The listing builds one solid part. Answer for the finished solid, in the listing's coordinates (mm). A direction names the side the tool comes from. Coordinates: 2 decimals unless noted, no trailing zeros. Loops run counter-clockwise (first coordinate to the right, second up) from the corner with the lowest first, then second, coordinate; pieces in that order, holes last. Notation, with made-up numbers: M -7,-21.75 L 17,-21.75 A9 ccw 17,-14.75 Z; hole C 14.25,75.5 d2. An arc over 180 degrees is marked long. Answer as a JSON object with one key per item and string values. Group by question number.
1. A cutting plane is placed at C-C on z = -26.1. Give the vertices of the cut face in (x, y), and give its area (3 significant figures).
2. Determine the mould class of faces 1 (the face through (-4, 1, -20.6)), 2 (the face through (7, 3.95, -26)), 3 (the face through (-20.45, 7.89, -25.22)) for opening direction Z: released by +Z, released by -Z, zero draft, split by the parting line, or undercut.
3. A cutting plane is placed at B-B on z = -19.5. Give the vertices of the cut face in (x, y), and give its area (3 significant figures).
4. A cutting plane is placed at A-A on x = -21.6. Give the vertices of the cut face in (y, z).
5. For faces 4 (the face through (-7.45, 6.43, -15.73)), 5 (the face through (32.72, 7.55, -7.22)), 6 (the face through (-14.071, 3, -9)), 7 (the face through (-4, -2.85, -16)), determine the directions among +Z, -Z, +X, -X, +Y, -Y from which every point of the face is accessible in a straight line to the end or side of a thin tool.
6. A cutting plane is placed at D-D on y = -1.5. Give the vertices of the cut face in (x, z), and give its area (3 significant figures).
7. Straight lines are drawn through the part: L1, parallel to Z at x = -4, y = 8.75; L2, parallel to X at y = 4, z = -9; L3, parallel to Z at x = -21.6, y = 6.25. For each, find the intervals that lie inside material, in ascending order.
8. Given pin 1 (2.5 mm diameter, centred on x = -6.5, z = -28.5, fed in from -Y); pin 2 (2 mm diameter, centred on x = -7.5, y = 1, fed in from -Z); pin 3 (11 mm diameter, centred on x = -12, z = -17, fed in from -Y), each flat-ended and moving along its own axis, determine where each tip first touches the part or whether it passes through.
Autodesk Inventor part; units mm, degrees
ref_plane "Arbeitsebene8" through (22.1204, -2.15, -7.2) normal (1, 0, 0) x (0, 1, 0)
ref_plane "Arbeitsebene9" through (-36.7921, -9.8415, -30.1125) normal (-0.7071, 0, 0.7071) x (0.7071, 0, 0.7071)
ref_plane "Arbeitsebene11" through (-36.7921, -9.8415, -30.1125) normal (-0.7071, 0, 0.7071) x (0.7071, 0, 0.7071)
ref_plane "Arbeitsebene6" through (18.9, 3.95, -31.1) normal (0, 1, 0) x (-1, 0, 0)
sketch "Skizze13" plane through (18.9, 3.95, -31.1) normal (0, 1, 0) x (-1, 0, 0)
  circle A0 centre (40.5, 5) radius 1.45
  line L0 (29.1796, 0.9) -> (29.1796, 0)
  line L1 (45.5, 0) -> (29.1796, 0)
  line L2 (45.5, 0) -> (45.5, 10)
  line L3 (45.5, 10) -> (29.1796, 10)
  line L4 (29.1796, 10) -> (29.1796, 6.8717)
  line L5 (29.1796, 6.8717) -> (32.9296, 6.8717)
  line L6 (32.9296, 6.8717) -> (32.9296, 0.9)
  line L7 (32.9296, 0.9) -> (29.1796, 0.9)
  line L8 (24.1796, 0) -> (24.1796, 0.9)
  line L9 (24.1796, 0.9) -> (20.4296, 0.9)
  line L10 (20.4296, 0.9) -> (20.4296, 6.8717)
  line L11 (20.4296, 6.8717) -> (24.1796, 6.8717)
  line L12 (24.1796, 6.8717) -> (24.1796, 10)
  line L13 (24.1796, 10) -> (0, 10)
  line L14 (0, 0) -> (0, 10)
  line L15 (24.1796, 0) -> (0, 0)
  circle A1 centre (14.9199, 5) radius 1.45
  circle A2 centre (5.0801, 5) radius 1.45
  line L16 (29.1796, 10) -> (24.1796, 10)
  line L17 (29.1796, 0) -> (24.1796, 0)
  line L18 (55.5, 0) -> (55.5, 10)
  line L19 (55.5, 10) -> (55.473, 10)
  line L20 (55.473, 10) -> (55.473, 40)
  line L21 (55.473, 40) -> (45.5, 40)
  line L22 (45.5, 40) -> (45.5, 20)
  line L23 (45.5, 20) -> (35.5, 20)
  line L24 (35.5, 20) -> (35.5, 10.0274)
  arc A3 (35.5, 10.0274) -> (35.527, 10) centre (40.5, 14.9264) ccw
  line L25 (45.5, 10) -> (35.527, 10)
  line L26 (45.5, 0) -> (45.5, 10)
  line L27 (45.5, 0) -> (55.5, 0)
  line L28 (52.073, 16.5) -> (52.073, 3.5)
  arc A4 (48.873, 3.5) -> (52.073, 3.5) centre (50.473, 3.5) ccw
  line L29 (48.873, 3.5) -> (48.873, 16.5)
  arc A5 (52.073, 16.5) -> (48.873, 16.5) centre (50.473, 16.5) ccw
  line L30 (48.8865, 23.1111) -> (48.8865, 36.1111)
  arc A6 (52.0865, 36.1111) -> (48.8865, 36.1111) centre (50.4865, 36.1111) ccw
  line L31 (52.0865, 36.1111) -> (52.0865, 23.1111)
  arc A7 (48.8865, 23.1111) -> (52.0865, 23.1111) centre (50.4865, 23.1111) ccw
  line L32 (-10, 0) -> (0, 0)
  line L33 (0, 10) -> (0, 0)
  line L34 (16, 10) -> (0, 10)
  line L35 (16, 10) -> (16, 20)
  line L36 (16, 20) -> (-10, 20)
  line L37 (-10, 20) -> (-10, 0)
  line L38 (-3.4, 16.5) -> (-3.4, 3.5)
  arc A8 (-6.6, 3.5) -> (-3.4, 3.5) centre (-5, 3.5) ccw
  line L39 (-6.6, 3.5) -> (-6.6, 16.5)
  arc A9 (-3.4, 16.5) -> (-6.6, 16.5) centre (-5, 16.5) ccw
  line L40 (-16.2879, 40) -> (45.5, 40)
  line L41 (45.5, 40) -> (45.5, 20.5)
  line L42 (45.5, 20.5) -> (-16.2879, 20.5)
  line L43 (-16.2879, 20.5) -> (-16.2879, 40)
  line L44 (45.5, 20.5) -> (35.5, 20.5)
  line L45 (35.5, 20.5) -> (35.5, 20)
  line L46 (35.5, 20) -> (45.5, 20)
  line L47 (45.5, 20) -> (45.5, 20.5)
  line L48 (16, 20) -> (0, 20)
  line L49 (0, 20) -> (0, 20.5)
  line L50 (0, 20.5) -> (16, 20.5)
  line L51 (16, 20.5) -> (16, 20)
  line L52 (0, 20) -> (0, 10)
  line L53 (35.5, 10) -> (45.5, 10)
  line L54 (45.5, 10) -> (45.5, 20.5)
  line L55 (45.5, 20.5) -> (35.5, 20.5)
  line L56 (35.5, 20.5) -> (35.5, 10)
  point P0 (0, 20)
  point P1 (0.5252, 10)
  point P2 (35.527, 10)
  point P3 (0, 20)
  point P4 (35.5, 10.0274)
  dimension "d60" = 0.5
extrude "Extrusion12" add sketch "Skizze13" along normal blind 8 contours L7 L6 L5 L4 L3 L2 L1 L0 | L0 L17 L8 L9 L10 L11 L12 L16 L4 L5 L6 L7 | L15 L14 L13 L12 L11 L10 L9 L8 | L3 A3 L24 L23 L54 | L23 L45 L42 L22 | L52 L36 L35 L13 | L16 L13 L35 L51 L42 L45 L24 L56 L3 | L42 L43 L40 L22 | L49 L42 L51 L36
sketch "Skizze16" plane through (18.9, 3.95, -31.1) normal (0, -1, 0) x (1, 0, 0)
  line L0 (16.2879, 20.5) -> (0, 20.5)
  line L1 (-45.5, 0) -> (-45.5, 40)
  circle A0 centre (-5.0801, 5) radius 1.45
  circle A1 centre (-14.9199, 5) radius 1.45
  line L2 (-16, 20) -> (10, 20)
  line L3 (-66.9798, -10.3003) -> (9.2505, 65.9301)
  line L4 (16.2879, 20.5) -> (0, 20.5)
  line L5 (16.2879, 20.5) -> (-45.5, 20.5)
  line L6 (-45.5, 20.5) -> (-45.5, 40)
  line L7 (-45.5, 40) -> (16.2879, 40)
  line L8 (16.2879, 40) -> (16.2879, 20.5)
  line L9 (0, 20.5) -> (0, 0)
  line L10 (16.2879, 40) -> (16.2879, 20.5)
  line L11 (-45.5, 40) -> (16.2879, 40)
  line L12 (0, 0) -> (-45.5, 0)
  point P0 (-18.9, 31.1)
extrude "Extrusion13" add sketch "Skizze16" along normal blind 8 contours L0 L5 L3 L7 L8 | L5 L1 L7 L3
ref_plane "Arbeitsebene7" through (-7.7796, -1.85, -37.9251) normal (1, 0, 0) x (0, -1, 0)
sketch "Skizze18" plane through (-7.7796, -1.85, -37.9251) normal (1, 0, 0) x (0, -1, 0)
  arc A0 (-5.8, -13.6968) -> (-0.7, -9.8391) centre (-5.8, -8.3968) ccw
  line L0 (-0.7, -9.8391) -> (-0.7, -7.7251)
  arc A1 (-10.8, -9.8251) -> (-0.8, -9.8251) centre (-5.8, -8.3968) ccw
  line L1 (-0.8, -7.8251) -> (-0.8, -9.8251)
  line L2 (-10.8, -7.8251) -> (-0.8, -7.8251)
  line L3 (-10.8, -9.8251) -> (-10.8, -7.8251)
  arc A2 (-10.9, -9.8391) -> (-0.7, -9.8391) centre (-5.8, -8.3968) ccw
  line L4 (-10.9, -9.8391) -> (-10.9, -7.7251)
  line L5 (-10.9, -7.7251) -> (-0.7, -7.7251)
  line L6 (-0.7, -7.7251) -> (-0.7, -9.8391)
  point P0 (-1.85, -37.9251)
  point P1 (-5.8, -13.6968)
extrude "Extrusion15" cut sketch "Skizze18" along normal mid plane 12.5 contours A2 L4 L5 L0 A0 | L3 L2 L1 A1
sketch "Skizze19" plane through (35.1879, 11.95, 8.9) normal (1, 0, 0) x (0, 0, -1)
  circle A0 centre (10, -8) radius 7
  circle A1 centre (10, -8) radius 7.1
  line L0 (14.0992, -15.1) -> (5.9008, -15.1)
  line L1 (5.9008, -15.1) -> (1.8016, -8)
  line L2 (1.8016, -8) -> (5.9008, -0.9)
  line L3 (5.9008, -0.9) -> (14.0992, -0.9)
  line L4 (14.0992, -0.9) -> (18.1984, -8)
  line L5 (18.1984, -8) -> (14.0992, -15.1)
  line L6 (19.5, -16) -> (0, -16)
  point P0 (8.9, -11.95)
  dimension "d68" = 0.1
ref_plane "Arbeitsebene8" through (22.1204, -2.15, -7.2) normal (1, 0, 0) x (0, 1, 0)
extrude "Extrusion16" cut sketch "Skizze19" against normal blind 5 contours A0 | A1 | A1 L4 L5 | A1 L3 L4 | L5 L0 A1 | A1 L2 L3 | L0 L1 A1 | A1 L1 L2
sketch "Skizze20" plane through (30.1879, 11.05, 2.9992) normal (1, 0, 0) x (0, 0, -1)
  arc A0 (6.1223, -12.104) -> (2.4773, -12.2481) centre (4.0992, -7.1) ccw
  circle A1 centre (4.0992, -7.1) radius 6.15
  line L0 (10.2492, -7.1) -> (-2.0508, -7.1)
  line L1 (-2.0508, -7.1) -> (-2.0508, -16.2052)
  line L2 (-2.0508, -16.2052) -> (10.2492, -16.2052)
  line L3 (10.2492, -16.2052) -> (10.2492, -7.1)
  point P0 (2.9992, -11.05)
  point P1 (-2.0508, -7.1)
  dimension "d71" = 12.3
ref_plane "Arbeitsebene9" through (-36.7921, -9.8415, -30.1125) normal (-0.7071, 0, 0.7071) x (0.7071, 0, 0.7071)
extrude "Extrusion17" cut sketch "Skizze20" against normal up to surface surface through (-36.7921, -9.8415, -30.1125) normal (-0.7071, 0, 0.7071)
ref_plane "Arbeitsebene10" through (13.1879, 11.05, 2.9992) normal (-1, 0, 0) x (0, 0, 1)
sketch "Skizze21" plane through (13.1879, 11.05, 2.9992) normal (-1, 0, 0) x (0, 0, 1)
  arc A0 (-3.1969, -9.9981) -> (-5.2274, -9.9178) centre (-4.0992, -7.1) ccw
  circle A1 centre (-4.0992, -7.1) radius 9
  line L0 (-13.0992, -7.1) -> (4.9008, -7.1)
  line L1 (4.9008, -7.1) -> (4.9008, -20.07)
  line L2 (4.9008, -20.07) -> (-13.0992, -20.07)
  line L3 (-13.0992, -20.07) -> (-13.0992, -7.1)
  point P0 (-2.9992, -11.05)
  dimension "d75" = 18
ref_plane "Arbeitsebene11" through (-36.7921, -9.8415, -30.1125) normal (-0.7071, 0, 0.7071) x (0.7071, 0, 0.7071)
extrude "Extrusion18" cut sketch "Skizze21" along normal up to surface surface through (-36.7921, -9.8415, -30.1125) normal (-0.7071, 0, 0.7071)
sketch "Skizze22" plane through (18.9, -4.05, -31.1) normal (0, -1, 0) x (1, 0, 0)
  line L0 (-45.5, 20.5) -> (16.2879, 20.5)
  line L1 (-45.5, 40) -> (-45.5, 20.5)
  line L2 (-34.6684, 23.7083) -> (-19.8191, 38.5575)
  line L3 (-19.8191, 38.5575) -> (-18.9706, 37.709)
  line L4 (-18.9706, 37.709) -> (-33.8198, 22.8597)
  line L5 (-33.8198, 22.8597) -> (-34.6684, 23.7083)
  line L6 (-34.6684, 23.7083) -> (-18.9706, 37.709) construction
  line L7 (-19.8191, 38.5575) -> (-33.8198, 22.8597) construction
  line L8 (-34.6684, 23.7083) -> (-13.6684, 23.7083) construction
  line L9 (16.2879, 40) -> (-45.5, 40)
  line L10 (16.2879, 20.5) -> (16.2879, 40)
  point P0 (-18.9, 31.1)
  point P1 (-26.8195, 30.7086)
  dimension "d78" = 21
  dimension "d79" = 45
  dimension "d80" = 1.2
extrude "Extrusion19" cut sketch "Skizze22" against normal blind 14 contours L2 L3 L4 L5
sketch "Skizze23" plane through (18.9, -4.05, -31.1) normal (0, -1, 0) x (1, 0, 0)
  line L0 (-45.5, 20.5) -> (16.2879, 20.5)
  line L1 (-45.5, 40) -> (-45.5, 20.5)
  line L2 (-35.6796, 21) -> (-32.9713, 23.7083)
  line L3 (-33.3878, 23.2918) -> (-30.8027, 25.8769)
  line L4 (-5.7121, 21) -> (-35.6796, 21)
  line L5 (-32.9713, 21) -> (-32.9713, 23.7083)
  line L6 (-18.9706, 37.709) -> (-19.9714, 36.7082)
  line L7 (-19.9714, 36.7082) -> (-17.0744, 36.7082)
  line L8 (-17.0744, 36.7082) -> (-17.0744, 39)
  line L9 (-18.9706, 37.709) -> (-19.9714, 36.7082)
  line L10 (-19.9714, 36.7082) -> (-17.6796, 39)
  line L11 (-17.6796, 39) -> (-17.0744, 39)
  line L12 (16.2879, 40) -> (-45.5, 40)
  line L13 (16.2879, 20.5) -> (16.2879, 40)
  point P0 (-18.9, 31.1)
  point P1 (-29.1796, 21)
extrude "Extrusion20" add sketch "Skizze23" against normal up to surface (16 mm away) contours L2 L5 L4 | L10 L11 L8 L7 L6
sketch "Skizze24" plane through (30.1879, 11.95, 8.9) normal (1, 0, 0) x (0, 0, -1)
  arc A0 (16.15, -8) -> (3.85, -8) centre (10, -8) ccw
  circle A1 centre (10, -8) radius 2.5
  circle A2 centre (10, -8) radius 6.15
  line L0 (14.0992, -0.9) -> (18.1984, -8)
  line L1 (18.1984, -8) -> (14.0992, -15.1)
  line L2 (14.0992, -15.1) -> (5.9008, -15.1)
  line L3 (5.9008, -15.1) -> (1.8016, -8)
  line L4 (1.8016, -8) -> (5.9008, -0.9)
  line L5 (5.9008, -0.9) -> (14.0992, -0.9)
  line L6 (19.5, -16) -> (19.5, 0)
  line L7 (0, 0) -> (19.5, 0)
  line L8 (0, -16) -> (0, 0)
  line L9 (19.5, -16) -> (0, -16)
  point P0 (8.9, -11.95)
extrude "Extrusion21" add sketch "Skizze24" against normal blind 1 contours A2 A0 | L0 L1 L2 L3 L4 L5 | L9 L8 L7 L6
ref_plane "Arbeitsebene12" through (-26.6, -8.85, -11.1) normal (1, 0, 0) x (0, 1, 0)
sketch "Skizze25" plane through (18.9, 3.95, -10.6) normal (1, 0, 0) x (0, 0, -1)
  line L0 (0.5, -6.8) -> (20.5, -6.8)
  line L1 (0, -8) -> (0, 8)
  line L2 (0, 0) -> (10.5, 0)
  line L3 (0, 0) -> (10, 0)
  line L4 (10, 0) -> (10, -6.8)
  line L5 (10, -6.8) -> (0, -6.8)
  line L6 (0, -6.8) -> (0, 0)
  line L7 (10.5, 0) -> (10.5, -6.8)
  point P0 (-10.6, -3.95)
  point P1 (0, -6.8)
  dimension "d87" = 0.5
extrude "Extrusion22" add sketch "Skizze25" against normal up to surface (45.5 mm away) contours L5 L1 L2 L4 L0
sketch "Skizze26" plane through (18.9, 11.95, -31.1) normal (0, 0, -1) x (-1, 0, 0)
  line L0 (0, -8) -> (24.1796, -8)
  line L1 (0, 0) -> (24.1796, 0)
  line L2 (0, -8) -> (0, 0)
  line L3 (24.1796, -8) -> (29.1796, -8)
  circle A0 centre (26.6796, -8) radius 2.5
  line L4 (24.1796, -8) -> (24.1796, 0)
  point P0 (18.9, -11.95)
extrude "Extrusion23" cut sketch "Skizze26" against normal through all contours A0 L3 | L3 A0
properties part number "30_Lightsheet_generator_passive_lid_v0"
From the geometry:
{
 "1": {"outline": "M -26.6,3.95 L -23.05,3.95 L -23.05,11.95 L -26.6,11.95 Z; M -20.15,3.95 L -14.03,3.95 L -14.03,7.99 L -1.53,7.99 L -1.53,3.95 L 2.53,3.95 L 2.53,11.95 L -20.15,11.95 Z; M 5.43,3.95 L 12.37,3.95 L 12.37,11.95 L 5.43,11.95 Z; M 15.27,3.95 L 18.9,3.95 L 18.9,11.95 L 15.27,11.95 Z", "area": "244 mm²"},
 "2": {"face 1": "released by -Z", "face 2": "zero draft", "face 3": "undercut"},
 "3": {"outline": "M -26.6,-2.85 L 18.9,-2.85 L 18.9,11.95 L -26.6,11.95 Z; hole C -7.78,3.95 d5", "area": "654 mm²"},
 "4": {"outline": "M -4.05,-10.6 L -2.85,-10.6 L -2.85,-20.6 L 3.95,-20.6 L 3.95,-24.65 L 11.95,-24.65 L 11.95,8.9 L -4.05,8.9 Z; M 3.95,-31.1 L 11.95,-31.1 L 11.95,-27.55 L 3.95,-27.55 Z"},
 "5": {"face 4": "+Z, -Z", "face 5": "+X", "face 6": "-Y", "face 7": "-Z, +X, -X, -Y"},
 "6": {"outline": "M -26.6,-20.6 L 18.9,-20.6 L 18.9,-10.6 L 35.19,-10.6 L 35.19,-6.15 L 30.19,-6.15 L 30.19,3.95 L 35.19,3.95 L 35.19,8.9 L -26.6,8.9 Z; hole M -15.77,-7.39 L -14.92,-8.24 L -14.07,-7.39 L -14.07,-10.1 L 13.19,-10.1 L 13.19,-7.25 L 29.19,-7.25 L 29.19,5.05 L 13.19,5.05 L 13.19,7.9 L 1.83,7.9 L 1.83,5.61 L -1.07,5.61 L -0.07,6.61 L -0.92,7.46 Z", "area": "1,020 mm²"},
 "7": {"L1": "z = -31.1 to -30.2, -27.28 to -8.71, 4.38 to 8.9", "L2": "x = -26.6 to -14.07, 13.19 to 30.19", "L3": "z = -31.1 to -27.55, -24.65 to 8.9"},
 "8": {"pin 1": "stops at y = 8.74", "pin 2": "stops at z = -20.6", "pin 3": "stops at y = -2.85"}
}
